from build123d import *

# Parameters (mm, degrees)
SKETCH1_W           = 120
SKETCH1_H           = 120
SKETCH1_R           = 1.5
SKETCH1_W_2         = 5
SKETCH1_H_2         = 5
BOSS_EXTRUDE1_DEPTH = 5
FILLET1_R           = 5


with BuildPart() as part:
    # Sketch1 → Boss-Extrude1 (new body)
    with BuildSketch(Plane.XY):
        with Locations((60, 60)):
            Rectangle(SKETCH1_W, SKETCH1_H)
        with Locations((112.5, 60)):
            Circle(SKETCH1_R, mode=Mode.SUBTRACT)
        with Locations((7.5, 60)):
            Circle(SKETCH1_R, mode=Mode.SUBTRACT)
        with Locations((60, 112.5)):
            Circle(SKETCH1_R, mode=Mode.SUBTRACT)
        with Locations(Location((60, 7.5, 0), (0, 0, 90))):
            Circle(SKETCH1_R, mode=Mode.SUBTRACT)
        with Locations((112.5, 52.5)):
            Rectangle(SKETCH1_W_2, SKETCH1_H_2, mode=Mode.SUBTRACT)
        with Locations((112.5, 67.5)):
            Rectangle(SKETCH1_W_2, SKETCH1_H_2, mode=Mode.SUBTRACT)
        with Locations((7.5, 52.5)):
            Rectangle(SKETCH1_W_2, SKETCH1_H_2, mode=Mode.SUBTRACT)
        with Locations((7.5, 67.5)):
            Rectangle(SKETCH1_W_2, SKETCH1_H_2, mode=Mode.SUBTRACT)
        with Locations((67.5, 112.5)):
            Rectangle(SKETCH1_W_2, SKETCH1_H_2, mode=Mode.SUBTRACT)
        with Locations((52.5, 112.5)):
            Rectangle(SKETCH1_W_2, SKETCH1_H_2, mode=Mode.SUBTRACT)
        with Locations((67.5, 7.5)):
            Rectangle(SKETCH1_W_2, SKETCH1_H_2, mode=Mode.SUBTRACT)
        with Locations((52.5, 7.5)):
            Rectangle(SKETCH1_W_2, SKETCH1_H_2, mode=Mode.SUBTRACT)
    extrude(amount=BOSS_EXTRUDE1_DEPTH)

    # Fillet1
    fillet1_edges = [part.edges().sort_by_distance(p)[0] for p in [
        (0, 120, 2.5),
        (120, 120, 2.5),
        (120, 0, 2.5),
        (0, 0, 2.5),
    ]]
    fillet(fillet1_edges, radius=FILLET1_R)


solid = part.part
The listing builds one solid part. Answer for the finished solid, in the listing's coordinates (mm). A direction names the side the tool comes from. Round coordinates to 2 decimals unless told otherwise and drop trailing zeros. Write each loop counter-clockwise with the first axis right and the second up, starting at its lowest first coordinate (ties: lowest second). Pieces come first, ordered by that corner, then holes. Notation, with made-up numbers: (86, 38.5) - (131, 38.5) arc R21 ccw to (131, 77.5) - close; hole circle Ø4 at (-8, 72.25). An arc over 180 degrees is marked (long way). Use one line per item in the form item = value. Start each with the question number.
Item 1: A cutting plane is placed at A-A (x = 60). Write down the section's boundary in (y, z), plus the area to 3 significant figures.
Item 2: A tool of negligible diameter and unlimited length cuts with its end or side. For faces 4 (the flat face through (59, 0, 2)), 5 (the flat face through (67, 110, 2)), from which of +Z, -Z, +X, -X, +Y, -Y can it reach the whole face along a straight path? Write none if from no direction.
Item 3: Determine the mould class of faces 1 (the cylindrical face through (1, 2, 3)), 2 (the flat face through (0, 59, 2)), 3 (the flat face through (7, 55, 2)) for opening direction Y: +Y half, -Y half, draft (parallel to the pull), parting line (faces both ways), or undercut.
Item 4: Find the intervals of material crossed by line 1 (X direction, y = 112.5, z = 1.6); line 2 (Y direction, x = 53, z = 0.6); line 3 (Y direction, x = 60, z = 2.15), in increasing order. Write a range as [from, to].
Item 5: A cutting plane is placed at B-B (y = 7.5). Write down the section's boundary in (x, z), plus the area to 3 significant figures.
The answers:
q1.outline = (0, 0) - (6, 0) - (6, 5) - (0, 5) - close; (9, 0) - (111, 0) - (111, 5) - (9, 5) - close; (114, 0) - (120, 0) - (120, 5) - (114, 5) - close
q1.area = 570 mm^2
q2.face_4 = +Z, -Z, +X, -X, -Y
q2.face_5 = +Z, -Z
q3.face_1 = -Y half
q3.face_2 = draft
q3.face_3 = undercut
q4.line_1 = [0, 50], [55, 58.5], [61.5, 65], [70, 120]
q4.line_2 = [0, 5], [10, 110], [115, 120]
q4.line_3 = [0, 6], [9, 111], [114, 120]
q5.outline = (0, 0) - (50, 0) - (50, 5) - (0, 5) - close; (55, 0) - (58.5, 0) - (58.5, 5) - (55, 5) - close; (61.5, 0) - (65, 0) - (65, 5) - (61.5, 5) - close; (70, 0) - (120, 0) - (120, 5) - (70, 5) - close
q5.area = 535 mm^2
